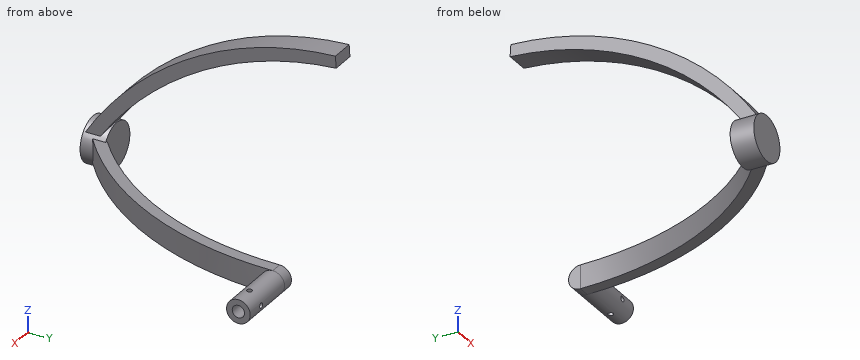
```python
from build123d import *

# Parameters (mm, degrees)
SKETCH1_R                = 5
BOSS_EXTRUDE1_DEPTH      = 25
SKETCH2_R                = 2.6
CUT_EXTRUDE1_DEPTH       = 25
CUT_EXTRUDE3_DEPTH       = 25
CUT_EXTRUDE3_DEPTH_BACK  = 25
SKETCH3_R                = 1.1
CUT_EXTRUDE4_DEPTH       = 25
CUT_EXTRUDE4_DEPTH_BACK  = 25
SKETCH4_R                = 1.1
BOSS_EXTRUDE2_DEPTH      = 5
BOSS_EXTRUDE2_DEPTH_BACK = 5
BOSS_EXTRUDE3_START      = 5
SKETCH6_R                = 5
BOSS_EXTRUDE3_DEPTH      = 5
BOSS_EXTRUDE4_DEPTH      = 5
BOSS_EXTRUDE4_DEPTH_BACK = 5
SKETCH8_R                = 9.5
BOSS_EXTRUDE10_DEPTH     = 10


with BuildPart() as part:
    # Sketch1 → Boss-Extrude1 (new body)
    with BuildSketch(Plane(origin=(0, 0, 0), x_dir=(0, 0, -1), z_dir=(1, 0, 0))):
        Circle(SKETCH1_R)
    extrude(amount=BOSS_EXTRUDE1_DEPTH)

    # Sketch2 → Cut-Extrude1 (cut)
    with BuildSketch(Plane.ZY):
        Circle(SKETCH2_R)
    extrude(amount=-CUT_EXTRUDE1_DEPTH, mode=Mode.SUBTRACT)

    # Sketch3 → Cut-Extrude3 (cut, two sides: drawn at the far end of the back side and taken through both)
    with BuildSketch(Plane(origin=(0, 0, 0), x_dir=(1, 0, 0), z_dir=(0, 1, 0)).offset(-CUT_EXTRUDE3_DEPTH_BACK)):
        with Locations(Location((17, 0, 0), (0, 0, 90))):
            Circle(SKETCH3_R)
    extrude(amount=CUT_EXTRUDE3_DEPTH + CUT_EXTRUDE3_DEPTH_BACK, mode=Mode.SUBTRACT)

    # Sketch4 → Cut-Extrude4 (cut, two sides: drawn at the far end of the back side and taken through both)
    with BuildSketch(Plane.XY.offset(-CUT_EXTRUDE4_DEPTH_BACK)):
        with Locations(Location((17, 0, 0), (0, 0, 180))):
            Circle(SKETCH4_R)
    extrude(amount=CUT_EXTRUDE4_DEPTH + CUT_EXTRUDE4_DEPTH_BACK, mode=Mode.SUBTRACT)



with BuildPart() as body_2:
    # Sketch5 → Boss-Extrude2 (new, two sides: drawn at the far end of the back side and taken through both)
    with BuildSketch(Plane.XY.offset(-BOSS_EXTRUDE2_DEPTH_BACK)):
        with BuildLine():
            Line((0, 0), (-5, 0))
            ThreePointArc((-5, 0), (-21.603552953, -63.499136863), (-67.164047662, -110.743815663))
            Line((-67.164047662, -110.743815663), (-58, -110.743815663))
            ThreePointArc((-58, -110.743815663), (-15.377599409, -62.506385089), (0, 0))
        make_face()
    extrude(amount=BOSS_EXTRUDE2_DEPTH + BOSS_EXTRUDE2_DEPTH_BACK)


with BuildPart() as part_1:
    add(part.part)

    add(body_2.part)  # Boss-Extrude3 merges body 2
    # Sketch6 → Boss-Extrude3 (add)
    with BuildSketch(Plane.ZY.offset(BOSS_EXTRUDE3_START)):
        with Locations(Location((0, 0, 0), (0, 0, 180))):
            Circle(SKETCH6_R)
    extrude(amount=-BOSS_EXTRUDE3_DEPTH)

    # Sketch7 → Boss-Extrude4 (add, two sides: drawn at the far end of the back side and taken through both)
    with BuildSketch(Plane(origin=(-58, -130.891746243, -8.226376206), x_dir=(0, 0.0627249424806172, -0.998030852023525), z_dir=(1, 0, 0)).offset(-BOSS_EXTRUDE4_DEPTH_BACK)):
        with BuildLine():
            Line((-68.071017976, 131.15), (-63.071017976, 131.15))
            ThreePointArc((-63.071017976, 131.15), (-46.774831734, 68.001453515), (-1.956245207, 20.624255297))
            Line((-1.956245207, 20.624255297), (-11.936553728, 20.93788001))
            ThreePointArc((-11.936553728, 20.93788001), (-53.801421124, 69.016374761), (-68.071017976, 131.15))
        make_face()
    extrude(amount=BOSS_EXTRUDE4_DEPTH + BOSS_EXTRUDE4_DEPTH_BACK)

    # Sketch8 → Boss-Extrude10 (add)
    with BuildSketch(Plane.XZ.offset(110.743815663)):
        with Locations(Location((-60.082023831, 0, 0), (0, 0, 270))):
            Circle(SKETCH8_R)
    extrude(amount=-BOSS_EXTRUDE10_DEPTH)


solid = part_1.part
```
Design review of the part built by this model. Coordinates are the model's own, in mm. Coordinates: 2 decimals unless noted, no trailing zeros. Loops run counter-clockwise (first coordinate to the right, second up) from the corner with the lowest first, then second, coordinate; pieces in that order, holes last. Notation, with made-up numbers: M 44.25,-15 L 53.25,-15 A29 ccw 53.25,6 Z; hole C -24.75,63 d3. An arc over 180 degrees is marked long. One line per question, with ' | ' between items.
(1) We need section C-C (y = -90.5). Give the boundary of the cut face in (x, z), and give its area (3 significant figures).
Filled in:
outline: M -63,22.46 L -53,22.46 L -53,30.52 L -63,30.52 Z; M -41.78,-5 L -34.92,-5 L -34.92,5 L -41.78,5 Z | area: 149 mm^2
(2) We need section B-B (x = 12.5). Give the boundary of the cut face in (y, z), and give its area (3 significant figures).
Filled in:
outline: C 0,0 d10; hole C 0,0 d5.2 | area: 57.3 mm^2
(3) Wall thickness on probe 1 along X at (y, z) = (3.7, 0); probe 2 along Y at (x, z) = (5, 0); probe 3 along X at (y, z) = (-100, 18): over which ranges is each line inside the solid? List them lowest first.
Filled in:
probe 1: x = -5 to 15.9, 18.1 to 25 | probe 2: y = -5 to -2.6, 2.6 to 5 | probe 3: x = -63 to -53
(4) For pin 1 Ø1.5 at (y, z) = (2, -2) entering from -X; pin 2 Ø19.5 at (x, z) = (-60.5, -3.5) entering from +Y; pin 3 Ø1.3 at (y, z) = (-2, 0.5) entering from +X; pin 4 Ø3 at (x, y) = (17, 0) entering from +Z, all flat-tipped, find the tip position at first contact; note any pin that passes through.
Filled in:
pin 1: stops at x = -5 | pin 2: stops at y = -98.88 | pin 3: stops at x = 25 | pin 4: stops at z = 5
(5) We need section A-A (y = -57). Give the boundary of the cut face in (x, z).
Filled in:
outline: M -63,47.95 L -53,47.95 L -53,54.35 L -63,54.35 Z; M -18.19,-5 L -12.65,-5 L -12.65,5 L -18.19,5 Z
(6) We need section D-D (z = 44.5). Give the boundary of the cut face in (x, y).
Filled in:
outline: M -63,-73.63 L -53,-73.63 L -53,-63.09 L -63,-63.09 Z
